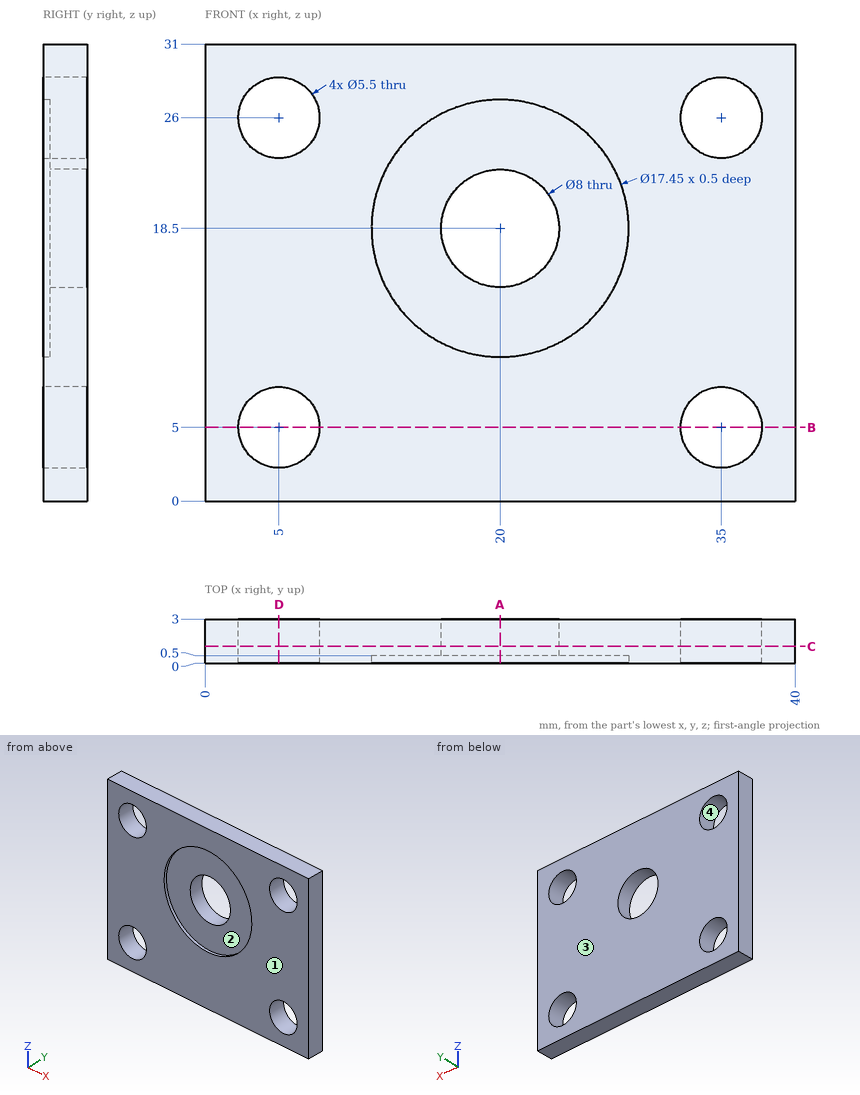
Check sheet for the drawn part. Datum: minimum x, y, z corner. Units: mm. A direction names the side the tool comes from. Coordinates: 2 decimals unless noted, no trailing zeros. Write each loop counter-clockwise with the first axis right and the second up, starting at its lowest first coordinate (ties: lowest second). Pieces come first, ordered by that corner, then holes. Notation, with made-up numbers: M 5.25,-37.5 L 56.25,-37.5 A7 ccw 56.25,-32.5 Z; hole C 74,17.25 d11. An arc over 180 degrees is marked long. Use a Markdown table: item, result.
Q1. Sectioned sample at D-D, the plane x = 5. Record the boundary of the cut face in (y, z), plus the area to 3 significant figures.
Reply:
| item | result |
|---|---|
| outline | M 0,0 L 3,0 L 3,2.25 L 0,2.25 Z; M 0,7.75 L 3,7.75 L 3,23.25 L 0,23.25 Z; M 0,28.75 L 3,28.75 L 3,31 L 0,31 Z |
| area | 60.0 mm² |
Q2. Set-up check for the marked faces 1 and 2: record each of +Z, -Z, +X, -X, +Y, -Y from which the full face is reachable in a straight line by a thin tool's end or side.
Reply:
| item | result |
|---|---|
| face 1 | +Z, -Z, +X, -X, -Y |
| face 2 | -Y |
Q3. Sectioned sample at B-B, the plane z = 5. Record the boundary of the cut face in (x, y).
Reply:
| item | result |
|---|---|
| outline | M 0,0 L 2.25,0 L 2.25,3 L 0,3 Z; M 7.75,0 L 32.25,0 L 32.25,3 L 7.75,3 Z; M 37.75,0 L 40,0 L 40,3 L 37.75,3 Z |
Q4. Sectioned sample at A-A, the plane x = 20. Record the boundary of the cut face in (y, z) (3 decimals).
Reply:
| item | result |
|---|---|
| outline | M 0,0 L 3,0 L 3,14.5 L 0.5,14.5 L 0.5,9.775 L 0,9.775 Z; M 0,27.225 L 0.5,27.225 L 0.5,22.5 L 3,22.5 L 3,31 L 0,31 Z |
Q5. Thickness scan on line 1 (X direction, y = 1.8, z = 26); line 2 (Z direction, x = 36.5, y = 0.6); line 3 (X direction, y = 2.8, z = 4). Record the ranges inside material, lowest first.
Reply:
| item | result |
|---|---|
| line 1 | x = 0 to 2.25, 7.75 to 32.25, 37.75 to 40 |
| line 2 | z = 0 to 2.7, 7.3 to 23.7, 28.3 to 31 |
| line 3 | x = 0 to 2.44, 7.56 to 32.44, 37.56 to 40 |
Q6. Go/stop test with flat-tipped pins: P1, Ø5, axis at x = 5, z = 26, coming from the +Y side; P2, Ø8.5, axis at x = 24, z = 20, coming from the -Y side. Record where each tip stops, or that it passes through.
Reply:
| item | result |
|---|---|
| P1 | passes through |
| P2 | stops at y = 0.5 |
Q7. Sectioned sample at C-C, the plane y = 1.15. Record the boundary of the cut face in (x, z), plus the area to 3 significant figures.
Reply:
| item | result |
|---|---|
| outline | M 0,0 L 40,0 L 40,31 L 0,31 Z; hole C 5,5 d5.5; hole C 5,26 d5.5; hole C 20,18.5 d8; hole C 35,5 d5.5; hole C 35,26 d5.5 |
| area | 1,090 mm² |
Q8. Draft check along X on the marked faces 3 and 4. Enter one of: +X half, -X half, draft (parallel to the pull), parting line (faces both ways), or undercut.
Reply:
| item | result |
|---|---|
| face 3 | draft |
| face 4 | undercut |
